from build123d import *

# Parameters (mm, degrees)
SKETCH2_R                       = 2.8194
SKETCH2_R_2                     = 1.5875
BOSS_EXTRUDE1_DEPTH             = 19.05
BOSS_EXTRUDE2_REACH             = 21.463
BOSS_EXTRUDE2_DIRECTION_2_REACH = 21.463
FILLET1_R                       = 2.54
SKETCH4_W                       = 6.5532
SKETCH4_H                       = 6.5532
CUT_EXTRUDE1_DEPTH              = 8.89
F_10_CLEARANCE_HOLE1_AT_2_COUNT = 2
F_10_CLEARANCE_HOLE1_AT_2_PITCH = 25.4


with BuildPart() as part:
    # Sketch2 → Boss-Extrude1 (new, symmetric)
    with BuildSketch(Plane.XY):
        with Locations(Location((0, 0, 0), (0, 0, 180))):
            Circle(SKETCH2_R)
        with Locations(Location((0, 0, 0), (0, 0, 180))):
            Circle(SKETCH2_R_2, mode=Mode.SUBTRACT)
    extrude(amount=BOSS_EXTRUDE1_DEPTH, both=True)

    # Boss-Extrude2: up to this face of the body (flat: up to its plane)
    boss_extrude2_end = Plane(part.part.faces().sort_by_distance((2.739655326, 0, 19.05))[0])
    # Sketch3 → Boss-Extrude2 (add, up to the picked face)
    with BuildSketch(Plane.XY, mode=Mode.PRIVATE) as boss_extrude2_sk1:
        with BuildLine():
            Line((2.662611866, -0.9271), (17.399, -0.9271))
            Line((17.399, -0.9271), (17.399, -2.2479))
            Line((17.399, -2.2479), (1.701752611, -2.2479))
            ThreePointArc((1.701752611, -2.2479), (2.279922692, -1.658604497), (2.662611866, -0.9271))
        make_face()
    boss_extrude2_tool1 = split(extrude(boss_extrude2_sk1.sketch, amount=BOSS_EXTRUDE2_REACH, mode=Mode.PRIVATE), bisect_by=boss_extrude2_end, keep=Keep.BOTH, mode=Mode.PRIVATE)
    add(boss_extrude2_tool1.solids().sort_by(Axis((9.838158, -1.594307, 0), (0, 0, 1)))[0])

    # Boss-Extrude2 direction 2: up to this face of the body (flat: up to its plane)
    boss_extrude2_direction_2_end = Plane(part.part.faces().sort_by_distance((2.739655326, 0, -19.05))[0])
    # Sketch3 → Boss-Extrude2 direction 2 (add, up to the picked face)
    with BuildSketch(Plane.XY, mode=Mode.PRIVATE) as boss_extrude2_direction_2_sk1:
        with BuildLine():
            Line((2.662611866, -0.9271), (17.399, -0.9271))
            Line((17.399, -0.9271), (17.399, -2.2479))
            Line((17.399, -2.2479), (1.701752611, -2.2479))
            ThreePointArc((1.701752611, -2.2479), (2.279922692, -1.658604497), (2.662611866, -0.9271))
        make_face()
    boss_extrude2_direction_2_tool1 = split(extrude(boss_extrude2_direction_2_sk1.sketch, amount=-BOSS_EXTRUDE2_DIRECTION_2_REACH, mode=Mode.PRIVATE), bisect_by=boss_extrude2_direction_2_end, keep=Keep.BOTH, mode=Mode.PRIVATE)
    add(boss_extrude2_direction_2_tool1.solids().sort_by(Axis((9.838158, -1.594307, 0), (0, 0, -1)))[0])

    # Fillet1
    fillet1_edges = [part.edges().sort_by_distance(p)[0] for p in [
        (1.701752611, -2.2479, 0),
    ]]
    fillet(fillet1_edges, radius=FILLET1_R)

    # Sketch4 → Cut-Extrude1 (cut, symmetric)
    with BuildSketch(Plane.XY):
        Rectangle(SKETCH4_W, SKETCH4_H)
    extrude(amount=CUT_EXTRUDE1_DEPTH, both=True, mode=Mode.SUBTRACT)

    # Sketch6 → #10 Clearance Hole1 (revolve, cut)
    with BuildSketch(Plane(origin=(11.049, -0.9271, -12.7), x_dir=(0, 0, 1), z_dir=(1, 0, 0))):
        Polygon((0, 0), (0, 1.8923), (2.8067, 1.8923), (2.8067, 0.635), (3.4417, 0), align=None)
    f_10_clearance_hole1 = revolve(axis=Axis((11.049, 5.4229, -12.7), (0, -1, 0)), mode=Mode.SUBTRACT)

    # #10 Clearance Hole1 at 2: #10 Clearance Hole1 ×2
    with Locations(*[(0, 0, i * F_10_CLEARANCE_HOLE1_AT_2_PITCH) for i in range(1, F_10_CLEARANCE_HOLE1_AT_2_COUNT)]):
        add(f_10_clearance_hole1, mode=Mode.SUBTRACT)


solid = part.part
Here's how the part is built. I have some questions about the finished solid (model axes, mm). A direction names the side the tool comes from. Round coordinates to 2 decimals unless told otherwise and drop trailing zeros. Order: outer loops, then holes, each group sorted by start corner. A loop starts at its lowest first (then second) coordinate and runs counter-clockwise, first axis right, second up. Notation, with made-up numbers: M 47.5,17 L 93.5,17 A32 ccw 93.5,51 Z; hole C 67,84 d7. An arc over 180 degrees is marked long. Return JSON: item names as keys, results as strings. Group by question number.
1. If we section it at D-D on x = 7: List the corners of the cut face in (y, z) for me, then the cut area to 3 significant figures.
2. If we section it at A-A on y = 0: List the corners of the cut face in (x, z) for me, then the cut area to 3 significant figures.
3. Please list where these lines run through material, in increasing order: probe 1 along Y at (x, z) = (0, 14); probe 2 along Z at (x, y) = (-1.5, -2); probe 3 along X at (y, z) = (0.1, -12.5).
4. If we mould it in two halves opening along X, with no side actions, what happens to faces 1 (the face through (1.83, -2.315, 14.041)), 2 (the face through (-0.73, 1.41, -14.04)), 3 (the face through (2, -1, -8.89))? For each: pulls with the +X half, pulls with the -X half, needs draft (parallel to the pull), parting line crosses it, or undercut.
5. If we section it at B-B on z = 12.7: List the corners of the cut face in (x, y) for me (1 decimal).
6. I'm going to push flat-ended pins straight in: pin 1 Ø1 at (y, z) = (-1.5, -2.5) entering from -X; pin 2 Ø4.5 at (x, z) = (7, 2) entering from +Y; pin 3 Ø1.5 at (y, z) = (1.5, 11.5) entering from +X. Where does each tip first touch, or does it pass through?
7. On a 3-axis mill with a long thin cutter (end or side, diameter ignored), from which of +Z, -Z, +X, -X, +Y, -Y can I reach the whole of each face in a straight line? I mean faces 4 (the face through (3.277, -2, 0)), 5 (the face through (10, -2.248, 0)), 6 (the face through (-0.73, 1.41, 13.9)). Say none if no direction works.
Reply:
{
 "1": {"outline": "M -2.25,-19.05 L -0.93,-19.05 L -0.93,19.05 L -2.25,19.05 Z", "area": "50.3 mm^2"},
 "2": {"outline": "M -2.82,-19.05 L -1.59,-19.05 L -1.59,-8.89 L -2.82,-8.89 Z; M -2.82,8.89 L -1.59,8.89 L -1.59,19.05 L -2.82,19.05 Z; M 1.59,-19.05 L 2.82,-19.05 L 2.82,-8.89 L 1.59,-8.89 Z; M 1.59,8.89 L 2.82,8.89 L 2.82,19.05 L 1.59,19.05 Z", "area": "50.1 mm^2"},
 "3": {"probe 1": "-2.82 to -1.59, 1.59 to 2.82", "probe 2": "-19.05 to -8.89, 8.89 to 19.05", "probe 3": "-2.82 to -1.58, 1.58 to 2.82"},
 "4": {"face 1": "pulls with the +X half", "face 2": "undercut", "face 3": "needs draft"},
 "5": {"outline": "M 1.3,-2.5 A2.5 cw 2.4,-2.2 L 8.2,-2.2 L 8.2,-1.6 L 7.6,-0.9 L 2.7,-0.9 A2.8 ccw long Z; M 13.9,-2.2 L 17.4,-2.2 L 17.4,-0.9 L 14.5,-0.9 L 13.9,-1.6 Z; hole C 0,0 d3.2"},
 "6": {"pin 1": "x = 3.28", "pin 2": "y = -0.93", "pin 3": "x = 2.72"},
 "7": {"face 4": "-X, +Y, -Y", "face 5": "+Z, -Z, +X, -Y", "face 6": "+Z, -Z"}
}
